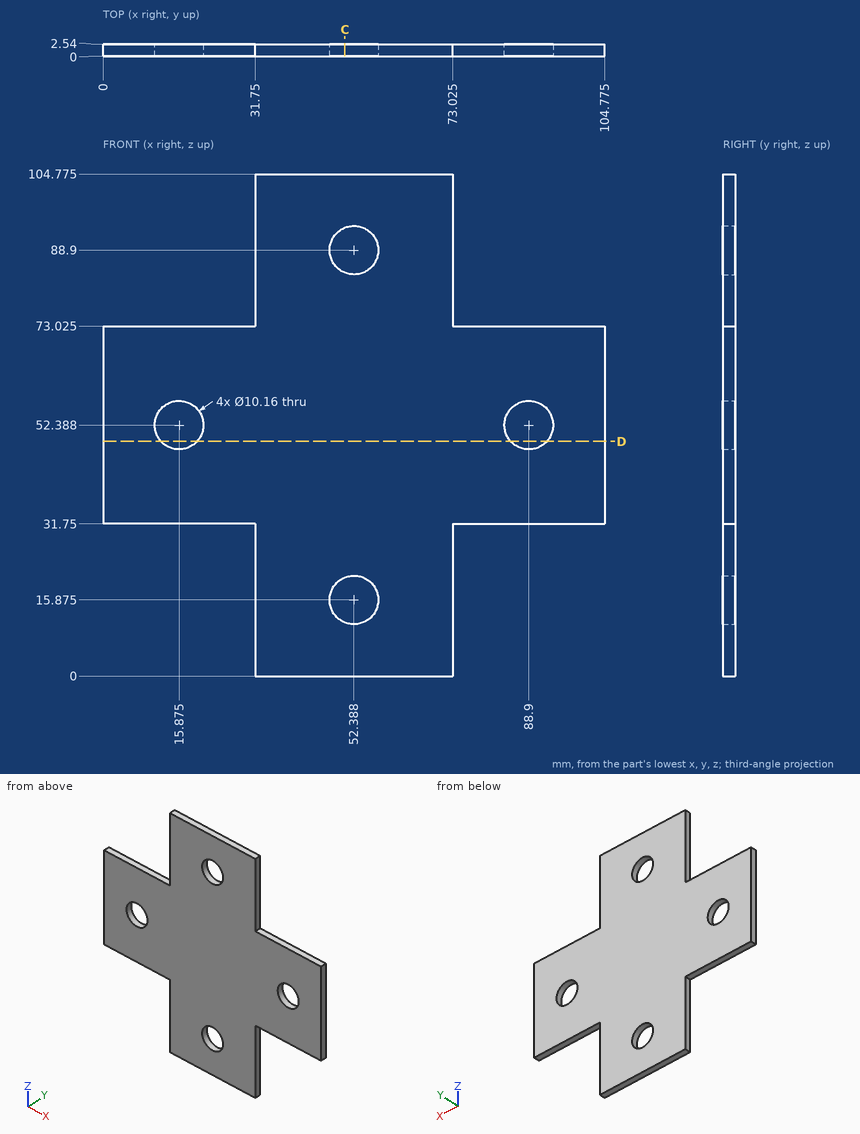
Can you work these out from the drawing? Everything is in mm from the part's minimum corner. Give positions to 0.01 mm unless a question says otherwise; leave off trailing zeros. Loops run counter-clockwise (first coordinate to the right, second up) from the corner with the lowest first, then second, coordinate; pieces in that order, holes last. Notation, with made-up numbers: (-4, -30) -> (38, -30) arc R3 ccw to (38, -26) -> close; hole circle Ø7 at (-6, 29). An arc over 180 degrees is marked (long way). Put each result on its own line as item: value.
(1) Please list where this line runs through material, in increasing order: probe 1 along Z at (x, y) = (56, 0.6) (1 decimal). Write a range as [from, to].
Computed:
probe 1: [0, 12.3], [19.4, 85.3], [92.5, 104.8]
(2) Imagine slicing it at D-D on z = 49. Write out the boundary of the cut face in (x, y) (1 decimal).
Computed:
outline: (0, 0) -> (12.1, 0) -> (12.1, 2.5) -> (0, 2.5) -> close; (19.7, 0) -> (85.1, 0) -> (85.1, 2.5) -> (19.7, 2.5) -> close; (92.7, 0) -> (104.8, 0) -> (104.8, 2.5) -> (92.7, 2.5) -> close
(3) Imagine slicing it at C-C on x = 50.5. Write out the boundary of the cut face in (y, z) (1 decimal), plus the area to 3 significant figures.
Computed:
outline: (0, 0) -> (2.5, 0) -> (2.5, 11.2) -> (0, 11.2) -> close; (0, 20.6) -> (2.5, 20.6) -> (2.5, 84.2) -> (0, 84.2) -> close; (0, 93.6) -> (2.5, 93.6) -> (2.5, 104.8) -> (0, 104.8) -> close
area: 218 mm^2
(4) I'm going to push flat-ended pins straight in: pin 1 Ø1.3 at (x, y) = (16.5, 2) entering from -Z; pin 2 Ø6 at (x, z) = (15.88, 52.39) entering from +Y; pin 3 Ø0.8 at (y, z) = (0.5, 90.5) entering from -X; pin 4 Ø0.8 at (y, z) = (1.5, 87) entering from +X (1 decimal). Where does each tip first touch, or does it pass through?
Computed:
pin 1: z = 31.75
pin 2: through
pin 3: x = 31.75
pin 4: x = 73
